For this review, take the finished solid that the model builds, in its own axes (mm). Coordinates: 2 decimals unless noted, no trailing zeros. Order: outer loops, then holes, each group sorted by start corner. A loop starts at its lowest first (then second) coordinate and runs counter-clockwise, first axis right, second up. Notation, with made-up numbers: (26, -20) -> (44, -20) arc R26 cw to (44, 5) -> close; hole circle Ø9 at (1.25, 78.25). An arc over 180 degrees is marked (long way). Return JSON: item names as keys, results as strings. Group by question number.
Item 1: Draft analysis for pull direction X (two halves, no side actions). For faces 1 (the flat face through (25.4, -41, 36)), 2 (the cylindrical face through (12.522, -40.367, 98.415)), 3 (the cylindrical face through (138.534, -51.901, 6.471)), state which applies: +X half, -X half, draft (parallel to the pull), parting line (faces both ways), or undercut.
Item 2: Take a section at A-A (z = 67.5). Write out the cut boundary in (x, y), then the cut area to 3 significant figures.
Item 3: Take a section at D-D (z = 41). Write out the cut boundary in (x, y), then the cut area to 3 significant figures.
Item 4: For line 1 along X through (y, z) = (-72, 18.5); line 2 along Z through (x, y) = (31, -29); line 3 along Z through (x, y) = (172, -48.5), list the stretches that pass through material, from the lowest coordinate up.
Item 5: Insertion check: pin 1 (1 mm diameter, centred on x = 164, y = -29.5, fed in from +Z). The pin has a flat end and moves straight along its axis. Give the tip position at first contact, or say it passes through.
Item 6: Take a section at B-B (y = -52). Write out the cut boundary in (x, z), then the cut area to 3 significant figures.
Item 7: Take a section at C-C (y = -17). Write out the cut boundary in (x, z).
```python
from build123d import *

# Parameters (mm, degrees)
F1_DEPTH = 82.55
F2_R     = 20.6375
F3_DEPTH = 152.4
F4_R     = 17.4625
F5_DEPTH = 25.4


with BuildPart() as f1:
    # F0 (on Front) → F1 (new body)
    with BuildSketch(Plane.XZ):
        Polygon((0, 114.3), (0, 0), (190.5, 0), (190.5, 12.7), (25.4, 12.9167754203), (25.4, 114.3), align=None)
    extrude(amount=F1_DEPTH)

    # F2 (on face) → F3 (cut)
    with BuildSketch(Plane(origin=(0, 0, 0), x_dir=(0, -1, 0), z_dir=(-1, 0, 0))):
        with Locations((41.275, 57.15)):
            Circle(F2_R)
        with BuildLine():
            Line((0, 114.3), (0, 57.15))
            ThreePointArc((0, 57.15), (41.275, 98.425), (82.55, 57.15))
            Line((82.55, 57.15), (82.55, 114.3))
            Line((82.55, 114.3), (0, 114.3))
        make_face()
    extrude(amount=-F3_DEPTH, mode=Mode.SUBTRACT)

    # F4 (on face) → F5 (cut)
    with BuildSketch(Plane(origin=(0.0170034164, 0, 12.9501031596), x_dir=(0.999999138, 0, -0.0013129935), z_dir=(0.0013129935, 0, 0.999999138))):
        with Locations((76.1831607755, -41.275)):
            Circle(F4_R)
        with Locations((152.3831607755, -41.275)):
            Circle(F4_R)
    extrude(amount=-F5_DEPTH, mode=Mode.SUBTRACT)


solid = f1.part
```
Findings below:
{
 "1": {"face 1": "+X half", "face 2": "draft", "face 3": "undercut"},
 "2": {"outline": "(0, -81.23) -> (25.4, -81.23) -> (25.4, -59.13) -> (0, -59.13) -> close; (0, -23.42) -> (25.4, -23.42) -> (25.4, -1.32) -> (0, -1.32) -> close", "area": "1,120 mm2"},
 "3": {"outline": "(0, -82.55) -> (25.4, -82.55) -> (25.4, -54.12) -> (0, -54.12) -> close; (0, -28.43) -> (25.4, -28.43) -> (25.4, 0) -> (0, 0) -> close", "area": "1,440 mm2"},
 "4": {"line 1": "x = 0 to 25.4", "line 2": "z = 0 to 12.91", "line 3": "z = 0 to 12.72"},
 "5": {"pin 1": "passes through"},
 "6": {"outline": "(0, 0) -> (62.4, 0) -> (62.42, 12.87) -> (25.4, 12.92) -> (25.4, 39.52) -> (0, 39.52) -> close; (0, 74.78) -> (25.4, 74.78) -> (25.4, 97.01) -> (0, 97.01) -> close; (89.96, 0) -> (138.6, 0) -> (138.62, 12.77) -> (89.98, 12.83) -> close; (166.16, 0) -> (190.5, 0) -> (190.5, 12.7) -> (166.18, 12.73) -> close", "area": "2,980 mm2"},
 "7": {"outline": "(0, 0) -> (190.5, 0) -> (190.5, 12.7) -> (25.4, 12.92) -> (25.4, 90.53) -> (0, 90.53) -> close"}
}
